For this review, take the finished solid that the model builds, in its own axes (mm). A direction names the side the tool comes from. Give positions to 0.01 mm unless a question says otherwise; leave off trailing zeros. Write each loop counter-clockwise with the first axis right and the second up, starting at its lowest first coordinate (ties: lowest second). Pieces come first, ordered by that corner, then holes. Notation, with made-up numbers: (1, 24.25) -> (8, 24.25) arc R27 ccw to (8, 62.25) -> close; hole circle Ø4 at (-33, 79). An arc over 180 degrees is marked (long way). Answer as CSV lines item,"result".
```python
from build123d import *

# Parameters (mm, degrees)
BOSS_EXTRUDE1_DEPTH = 11
FILLET1_R           = 4
FILLET2_R           = 2.5
SKETCH2_R           = 1.525
CUT_EXTRUDE1_DEPTH  = 11


with BuildPart() as part:
    # Sketch1 → Boss-Extrude1 (new body)
    with BuildSketch(Plane.XY):
        Polygon((-5.95, 0), (-5.95, 9.95), (5.95, 9.95), (5.95, 0), (8.65875, 0), (14.45, 0), (14.45, 2.6), (8.45, 2.6), (8.45, 12.45), (-8.45, 12.45), (-8.45, 2.6), (-14.45, 2.6), (-14.45, 0), (-8.65875, 0), align=None)
    extrude(amount=BOSS_EXTRUDE1_DEPTH)

    # Fillet1
    fillet1_edges = [part.edges().sort_by_distance(p)[0] for p in [
        (-14.45, 1.3, 0),
        (14.45, 1.3, 0),
        (14.45, 1.3, 11),
        (-14.45, 1.3, 11),
    ]]
    fillet(fillet1_edges, radius=FILLET1_R)

    # Fillet2
    fillet2_edges = [part.edges().sort_by_distance(p)[0] for p in [
        (-8.45, 12.45, 5.5),
        (8.45, 12.45, 5.5),
    ]]
    fillet(fillet2_edges, radius=FILLET2_R)

    # Sketch2 → Cut-Extrude1 (cut)
    with BuildSketch(Plane(origin=(0, 2.6, 0), x_dir=(1, 0, 0), z_dir=(0, 1, 0))):
        with Locations(Location((-11.45, -5.5, 0), (0, 0, 180))):
            Circle(SKETCH2_R)
        with Locations(Location((11.45, -5.5, 0), (0, 0, 180))):
            Circle(SKETCH2_R)
    extrude(amount=-CUT_EXTRUDE1_DEPTH, mode=Mode.SUBTRACT)


solid = part.part
```
Q1. Add section C-C (y = 5.25). Write out the cut boundary in (x, z).
Answer block:
outline,"(-8.45, 0) -> (-5.95, 0) -> (-5.95, 11) -> (-8.45, 11) -> close; (5.95, 0) -> (8.45, 0) -> (8.45, 11) -> (5.95, 11) -> close"
Q2. Add section A-A (y = 1.75). Write out the cut boundary in (x, z) (3 decimals), plus the area to 3 significant figures.
Answer block:
outline,"(-14.45, 4) arc R4 ccw to (-10.45, 0) -> (-5.95, 0) -> (-5.95, 11) -> (-10.45, 11) arc R4 ccw to (-14.45, 7) -> close; (5.95, 0) -> (10.45, 0) arc R4 ccw to (14.45, 4) -> (14.45, 7) arc R4 ccw to (10.45, 11) -> (5.95, 11) -> close; hole circle Ø3.05 at (-11.45, 5.5); hole circle Ø3.05 at (11.45, 5.5)"
area,"159 mm2"
Q3. For faces 1 (the flat face through (0, 9.95, 5)), 2 (the cylindrical face through (10.63, 1.318, 6.786)), 3 (the flat face through (8.45, 6, 5)), 4 (the flat face through (-10, 2.6, 4)), 5 (the flat face through (-14.45, 1, 5)), list the 3-axis set-ups (+Z, -Z, +X, -X, +Y, -Y) from which the entire face can be reached by the end or side of a thin tool; tool diameter is ignored.
Answer block:
face 1,"+Z, -Z, -Y"
face 2,"+Y, -Y"
face 3,"+Z, -Z, +X, +Y"
face 4,"+Z, -Z, -X, +Y"
face 5,"+Z, -Z, -X, +Y, -Y"
Q4. Add section B-B (z = 5.5). Write out the cut boundary in (x, y) (3 decimals), plus the area to 3 significant figures.
Answer block:
outline,"(-14.45, 0) -> (-12.975, 0) -> (-12.975, 2.6) -> (-14.45, 2.6) -> close; (-9.925, 0) -> (-5.95, 0) -> (-5.95, 9.95) -> (5.95, 9.95) -> (5.95, 0) -> (9.925, 0) -> (9.925, 2.6) -> (8.45, 2.6) -> (8.45, 9.95) arc R2.5 ccw to (5.95, 12.45) -> (-5.95, 12.45) arc R2.5 ccw to (-8.45, 9.95) -> (-8.45, 2.6) -> (-9.925, 2.6) -> close; (12.975, 0) -> (14.45, 0) -> (14.45, 2.6) -> (12.975, 2.6) -> close"
area,"105 mm2"
Q5. To check wall thickness, follow probe 1 along X at (y, z) = (6.5, 6.5); probe 2 along Y at (x, z) = (-2, 5); probe 3 along Y at (x, z) = (10.5, 0.75). State the ranges of each line that lie inside material, in increasing order. Write a range as [from, to].
Answer block:
probe 1,"x = [-8.45, -5.95], [5.95, 8.45]"
probe 2,"y = [9.95, 12.45]"
probe 3,"y = [0, 2.6]"
Q6. Draft analysis for pull direction Z (two halves, no side actions). For faces 6 (the flat face through (-0.1, 10.5, 0)), 7 (the flat face through (14.45, 1, 5)), 8 (the cylindrical face through (-10.3, 1.3, 6.5)), 9 (the cylindrical face through (13.309, 1.318, 9.797)), state which applies: released by +Z, released by -Z, zero draft, split by the parting line, or undercut.
Answer block:
face 6,"released by -Z"
face 7,"zero draft"
face 8,"undercut"
face 9,"released by +Z"
Q7. Add section D-D (x = 11.45). Write out the cut boundary in (y, z) (3 decimals).
Answer block:
outline,"(0, 0.127) -> (2.6, 0.127) -> (2.6, 3.975) -> (0, 3.975) -> close; (0, 7.025) -> (2.6, 7.025) -> (2.6, 10.873) -> (0, 10.873) -> close"
Q8. Clearance check with flat-ended pins moving along their axes: pin 1 (3 mm diameter, centred on x = 10.5, z = 7.5, fed in from +Y); pin 2 (3.5 mm diameter, centred on y = 8, z = 7, fed in from +X); pin 3 (3.5 mm diameter, centred on y = 4.5, z = 3, fed in from -X); pin 4 (1.8 mm diameter, centred on x = 11.45, z = 5.5, fed in from -Y). State where each tip first meets the part, or that it passes through.
Answer block:
pin 1,"stops at y = 2.6"
pin 2,"stops at x = 8.45"
pin 3,"stops at x = -8.45"
pin 4,"passes through"
